Check sheet for the drawn part. Datum: minimum x, y, z corner. Units: mm. Round coordinates to 2 decimals unless told otherwise and drop trailing zeros. Loops run counter-clockwise (first coordinate to the right, second up) from the corner with the lowest first, then second, coordinate; pieces in that order, holes last. Notation, with made-up numbers: (24, 51.5) - (41, 51.5) arc R10 cw to (41, 66.5) - close; hole circle Ø1 at (65.25, -28.5). An arc over 180 degrees is marked (long way). Use CSV: the item, a comma, the result in double quotes.
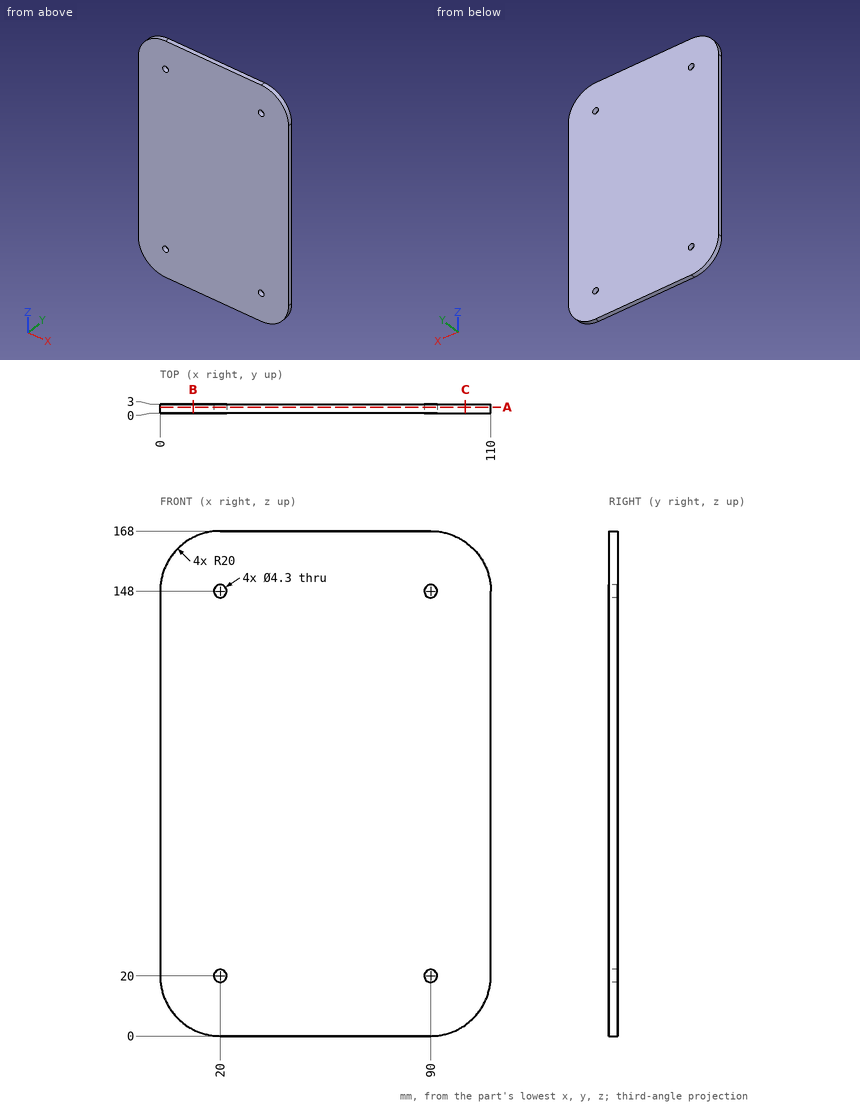
1) Cross-section at A-A, the plane y = 2. Record the cut outline in (x, z).
Returned:
outline,"(0, 20) arc R20 ccw to (20, 0) - (90, 0) arc R20 ccw to (110, 20) - (110, 148) arc R20 ccw to (90, 168) - (20, 168) arc R20 ccw to (0, 148) - close; hole circle Ø4.3 at (20, 20); hole circle Ø4.3 at (20, 148); hole circle Ø4.3 at (90, 20); hole circle Ø4.3 at (90, 148)"
2) Cross-section at B-B, the plane x = 11. Record the cut outline in (y, z), then the cut area to 3 significant figures.
Returned:
outline,"(0, 2.14) - (3, 2.14) - (3, 165.86) - (0, 165.86) - close"
area,"491 mm²"
3) Cross-section at C-C, the plane x = 101.5. Record the cut outline in (y, z), then the cut area to 3 significant figures.
Returned:
outline,"(0, 3.64) - (3, 3.64) - (3, 164.36) - (0, 164.36) - close"
area,"482 mm²"
4) Thickness scan on probe 1 along X at (y, z) = (1.2, 148); probe 2 along Z at (x, y) = (90, 2.05); probe 3 along Z at (x, y) = (10.5, 2.25). Record the ranges inside material, lowest first. Write a range as [from, to].
Returned:
probe 1,"x = [0, 17.85], [22.15, 87.85], [92.15, 110]"
probe 2,"z = [0, 17.85], [22.15, 145.85], [150.15, 168]"
probe 3,"z = [2.4, 165.6]"
